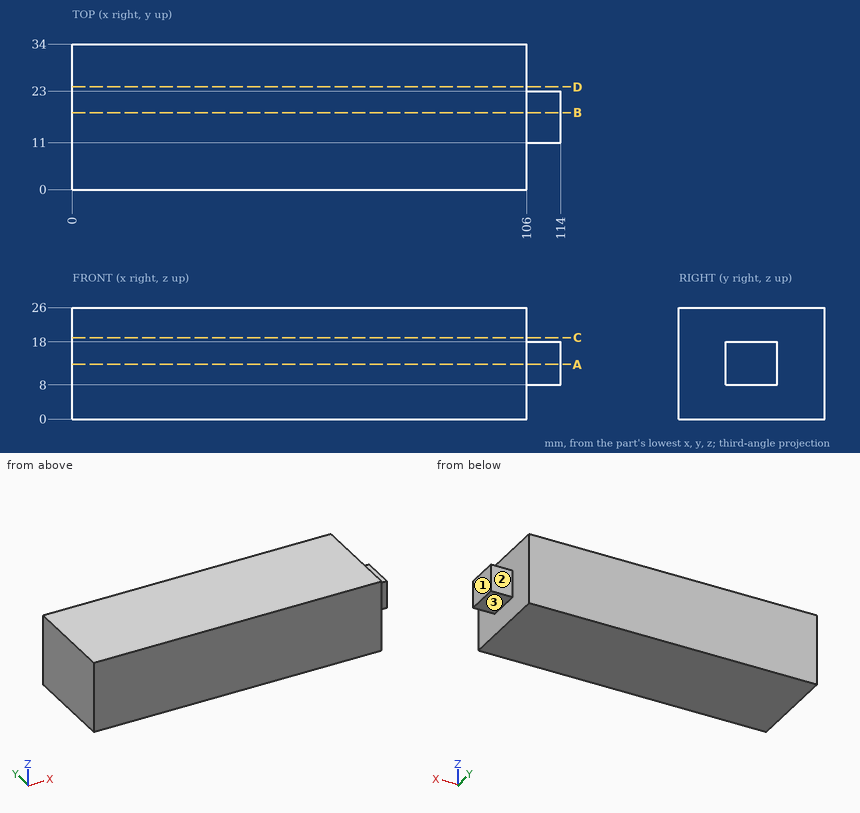
Job drawing, mm, ordinate dimensions from the low corner. One solid piece. A direction names the side the tool comes from. Coordinates: 2 decimals unless noted, no trailing zeros. Write each loop counter-clockwise with the first axis right and the second up, starting at its lowest first coordinate (ties: lowest second). Pieces come first, ordered by that corner, then holes. Notation, with made-up numbers: M 50.25,86 L 96.25,86 A13 ccw 96.25,94 Z; hole C -6,81 d11. An arc over 180 degrees is marked long. Answer as a JSON object with one key per item and string values. Group by question number.
1) Saw through at D-D (y = 24). Write the cut outline in (x, z).
2) Wall check: line 1 (X direction, y = 8, z = 18). Give the ranges that are in metal, low to high. Write a range as from..to.
3) Saw through at A-A (z = 12.75). Write the cut outline in (x, y), plus the area to 3 significant figures.
4) Saw through at B-B (y = 18). Write the cut outline in (x, z).
5) Tool access for the marked faces 1, 2 and 3: list every direction of +Z, -Z, +X, -X, +Y, -Y with a clear straight run to the whole face (end or side of a thin tool).
6) Pin check, flat tips, straight feed: pin 1 Ø9 at (x, z) = (111, 14.5) entering from -Y; pin 2 Ø4 at (x, y) = (108.5, 14) entering from -Z; pin 3 Ø4 at (y, z) = (29.5, 19.5) entering from +X. Stop position of each tip, or through.
7) Saw through at C-C (z = 19). Write the cut outline in (x, y).
Values follow:
{
 "1": {"outline": "M 0,0 L 106,0 L 106,26 L 0,26 Z"},
 "2": {"line 1": "x = 0..106"},
 "3": {"outline": "M 0,0 L 106,0 L 106,11 L 114,11 L 114,23 L 106,23 L 106,34 L 0,34 Z", "area": "3,700 mm2"},
 "4": {"outline": "M 0,0 L 106,0 L 106,8 L 114,8 L 114,18 L 106,18 L 106,26 L 0,26 Z"},
 "5": {"face 1": "+Z, -Z, +X, +Y, -Y", "face 2": "+Z, -Z, +X, +Y", "face 3": "-Z, +X, +Y, -Y"},
 "6": {"pin 1": "stops at y = 11", "pin 2": "stops at z = 8", "pin 3": "stops at x = 106"},
 "7": {"outline": "M 0,0 L 106,0 L 106,34 L 0,34 Z"}
}
